The listing builds one solid part. Answer for the finished solid, in the listing's coordinates (mm). Round coordinates to 2 decimals unless told otherwise and drop trailing zeros. Write each loop counter-clockwise with the first axis right and the second up, starting at its lowest first coordinate (ties: lowest second). Pieces come first, ordered by that corner, then holes.
(1) A cutting plane is placed at B-B, the plane y = -19. Give the vertices of the cut face in (x, z), and give its area (3 significant figures).
(2) Find the intervals of material crossed by probe 1 along X at (y, z) = (-17.5, -0.25); probe 2 along Y at (x, z) = (-45, 0.5); probe 3 along Y at (x, z) = (-22.5, 1), in increasing order.
(3) A cutting plane is placed at D-D, the plane x = -21. Give the vertices of the cut face in (y, z).
(4) A cutting plane is placed at C-C, the plane z = -3.5. Give the vertices of the cut face in (x, y), and give its area (3 significant figures).
(5) A cutting plane is placed at A-A, the plane x = -44.5. Give the vertices of the cut face in (y, z), and give its area (3 significant figures).
(6) Each of these flat-tipped pins is pushed along its axis until it touches: pin 1 Ø1.5 at (y, z) = (87, -1) entering from -X; pin 2 Ø3.5 at (y, z) = (-87, -2.5) entering from +X; pin 3 Ø2 at (x, y) = (14.5, 87) entering from -Z; pin 4 Ø3.5 at (x, z) = (-9, 0) entering from +Y. Where does it stop, or does it pass through?
from build123d import *

# Parameters (mm, degrees)
SKETCH1_W           = 111
SKETCH1_H           = 178
SKETCH1_W_2         = 101
SKETCH1_H_2         = 168
BOSS_EXTRUDE1_DEPTH = 6
SKETCH2_W           = 111
SKETCH2_H           = 178
SKETCH2_W_2         = 97
SKETCH2_H_2         = 155.54954955
BOSS_EXTRUDE2_DEPTH = 0.5
SKETCH3_W           = 60
SKETCH3_H           = 10
CUT_EXTRUDE1_DEPTH  = 77
SKETCH4_W           = 65
SKETCH4_H           = 10
CUT_EXTRUDE2_DEPTH  = 77
FILLET1_R           = 1
FILLET2_R           = 3
FILLET3_R           = 1


with BuildPart() as part:
    # Sketch1 → Boss-Extrude1 (new, symmetric)
    with BuildSketch(Plane.XY):
        Rectangle(SKETCH1_W, SKETCH1_H)
        Rectangle(SKETCH1_W_2, SKETCH1_H_2, mode=Mode.SUBTRACT)
    extrude(amount=BOSS_EXTRUDE1_DEPTH, both=True)

    # Sketch2 → Boss-Extrude2 (add, symmetric)
    with BuildSketch(Plane.XY.offset(6)):
        Rectangle(SKETCH2_W, SKETCH2_H)
        Rectangle(SKETCH2_W_2, SKETCH2_H_2, mode=Mode.SUBTRACT)
    extrude(amount=BOSS_EXTRUDE2_DEPTH, both=True)

    # Sketch3 → Cut-Extrude1 (cut)
    with BuildSketch(Plane.XZ.offset(-84)):
        with Locations((0, -1)):
            Rectangle(SKETCH3_W, SKETCH3_H)
    extrude(amount=-CUT_EXTRUDE1_DEPTH, mode=Mode.SUBTRACT)

    # Sketch4 → Cut-Extrude2 (cut)
    with BuildSketch(Plane(origin=(0, -84, 0), x_dir=(1, 0, 0), z_dir=(0, 1, 0))):
        with Locations((0, 6)):
            Rectangle(SKETCH4_W, SKETCH4_H)
    extrude(amount=-CUT_EXTRUDE2_DEPTH, mode=Mode.SUBTRACT)

    # Fillet1
    fillet1_edges = [part.edges().sort_by_distance(p)[0] for p in [
        (-48.5, -77.774774775, 6),
        (48.5, -77.774774775, 6),
        (48.5, 77.774774775, 6),
        (-48.5, 77.774774775, 6),
    ]]
    fillet(fillet1_edges, radius=FILLET1_R)

    # Fillet2
    # the kernel refuses this fillet: 3 mm, written as the material it takes off along each edge
    with BuildSketch(Plane(origin=(-52.5, -86, 3.5), x_dir=(0, -1, 0), z_dir=(0, 0, 1))) as fillet2_piece_1_section:
        Polygon((0, 0), (FILLET2_R, 0), (FILLET2_R, -FILLET2_R), (0, -FILLET2_R), align=None)
    fillet2_piece_1 = extrude(amount=FILLET2_R, mode=Mode.PRIVATE)
    fillet2_piece_1 = fillet2_piece_1 - Plane(origin=(-52.5, -86, 3.5), x_dir=(0.7071067811865475, 0.7071067811865477, 0), z_dir=(0, 0, 1)) * Sphere(FILLET2_R, mode=Mode.PRIVATE)
    add(fillet2_piece_1, mode=Mode.SUBTRACT)
    with BuildSketch(Plane(origin=(-52.5, 86, 3.5), x_dir=(-1, 0, 0), z_dir=(0, 0, 1))) as fillet2_piece_2_section:
        Polygon((0, 0), (FILLET2_R, 0), (FILLET2_R, -FILLET2_R), (0, -FILLET2_R), align=None)
    fillet2_piece_2 = extrude(amount=FILLET2_R, mode=Mode.PRIVATE)
    fillet2_piece_2 = fillet2_piece_2 - Plane(origin=(-52.5, 86, 3.5), x_dir=(0.7071067811865477, -0.7071067811865474, 0), z_dir=(0, 0, 1)) * Sphere(FILLET2_R, mode=Mode.PRIVATE)
    add(fillet2_piece_2, mode=Mode.SUBTRACT)
    with BuildSketch(Plane(origin=(52.5, -86, 3.5), x_dir=(0, -1, 0), z_dir=(0, 0, 1))) as fillet2_piece_3_section:
        Polygon((0, 0), (FILLET2_R, 0), (FILLET2_R, FILLET2_R), (0, FILLET2_R), align=None)
    fillet2_piece_3 = extrude(amount=FILLET2_R, mode=Mode.PRIVATE)
    fillet2_piece_3 = fillet2_piece_3 - Plane(origin=(52.5, -86, 3.5), x_dir=(-0.7071067811865476, 0.7071067811865475, 0), z_dir=(0, 0, 1)) * Sphere(FILLET2_R, mode=Mode.PRIVATE)
    add(fillet2_piece_3, mode=Mode.SUBTRACT)
    with BuildSketch(Plane(origin=(52.5, 86, 3.5), x_dir=(0, 1, 0), z_dir=(0, 0, 1))) as fillet2_piece_4_section:
        Polygon((0, 0), (FILLET2_R, 0), (FILLET2_R, -FILLET2_R), (0, -FILLET2_R), align=None)
    fillet2_piece_4 = extrude(amount=FILLET2_R, mode=Mode.PRIVATE)
    fillet2_piece_4 = fillet2_piece_4 - Plane(origin=(52.5, 86, 3.5), x_dir=(-0.7071067811865474, -0.7071067811865477, 0), z_dir=(0, 0, 1)) * Sphere(FILLET2_R, mode=Mode.PRIVATE)
    add(fillet2_piece_4, mode=Mode.SUBTRACT)
    with BuildSketch(Plane(origin=(-55.5, -86, 6.5), x_dir=(1, 0, 0), z_dir=(0, 1, 0)), Plane(origin=(55.5, 86, 6.5), x_dir=(-1, 0, 0), z_dir=(0, -1, 0))) as fillet2_piece_5:
        with BuildLine():
            CenterArc((FILLET2_R, FILLET2_R), FILLET2_R, 180, 90)
            Line((0, FILLET2_R), (0, 0))
            Line((0, 0), (FILLET2_R, 0))
        make_face()
    extrude(amount=172, mode=Mode.SUBTRACT)
    with BuildSketch(Plane(origin=(52.5, -89, 6.5), x_dir=(0, 1, 0), z_dir=(-1, 0, 0)), Plane(origin=(-52.5, 89, 6.5), x_dir=(0, -1, 0), z_dir=(1, 0, 0))) as fillet2_piece_6:
        with BuildLine():
            CenterArc((FILLET2_R, FILLET2_R), FILLET2_R, 180, 90)
            Line((0, FILLET2_R), (0, 0))
            Line((0, 0), (FILLET2_R, 0))
        make_face()
    extrude(amount=105, mode=Mode.SUBTRACT)
    with BuildSketch(Plane(origin=(55.5, 89, -13.5), x_dir=(-1, 0, 0), z_dir=(0, 0, 1))) as fillet2_piece_7:
        with BuildLine():
            CenterArc((FILLET2_R, FILLET2_R), FILLET2_R, 180, 90)
            Line((0, FILLET2_R), (0, 0))
            Line((0, 0), (FILLET2_R, 0))
        make_face()
    extrude(amount=17, mode=Mode.SUBTRACT)
    with BuildSketch(Plane(origin=(-55.5, 89, 3.5), x_dir=(0, -1, 0), z_dir=(0, 0, -1)), Plane(origin=(55.5, -89, -13.5), x_dir=(-1, 0, 0), z_dir=(0, 0, 1)), Plane(origin=(-55.5, -89, 3.5), x_dir=(1, 0, 0), z_dir=(0, 0, -1))) as fillet2_piece_8:
        with BuildLine():
            CenterArc((FILLET2_R, -FILLET2_R), FILLET2_R, 90, 90)
            Line((0, -FILLET2_R), (0, 0))
            Line((0, 0), (FILLET2_R, 0))
        make_face()
    extrude(amount=17, mode=Mode.SUBTRACT)

    # Fillet3
    fillet3_edges = [part.edges().sort_by_distance(p)[0] for p in [
        (-30, 89, -1.25),
        (-30, 88.989491568, 3.750878781),
        (30, 88.989491568, 3.750878781),
        (30, 89, -1.25),
        (-30, 84, -1),
        (30, 84, -1),
        (0, 84, 4),
        (0, -89, -1),
        (32.5, -89, -3.5),
        (-32.5, -89, -3.5),
        (32.5, -84, -3.5),
        (-32.5, -84, -3.5),
        (0, -84, -1),
    ]]
    fillet(fillet3_edges, radius=FILLET3_R)


solid = part.part
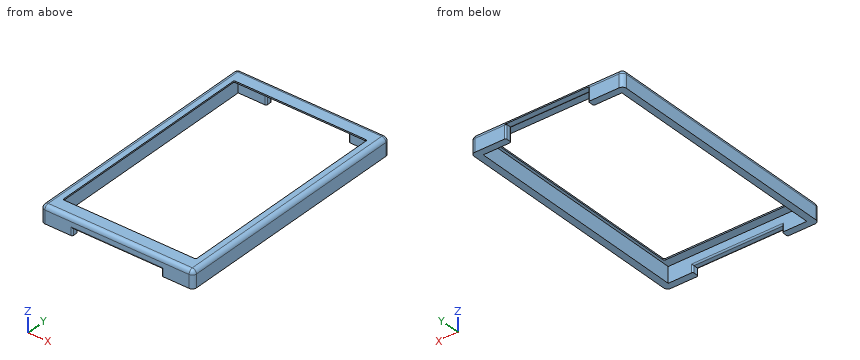
Solutions:
1. outline: (-55.5, -6) - (-50.5, -6) - (-50.5, 5.5) - (-48.5, 5.5) - (-48.5, 6.5) - (-52.5, 6.5) arc R3 ccw to (-55.5, 3.5) - close; (48.5, 5.5) - (50.5, 5.5) - (50.5, -6) - (55.5, -6) - (55.5, 3.5) arc R3 ccw to (52.5, 6.5) - (48.5, 6.5) - close
1. area: 125 mm2
2. probe 1: x = -55.5 to -50.5, 50.5 to 55.5
2. probe 2: y = -89 to -84, 84 to 89
2. probe 3: y = -89 to -84
3. outline: (-89, 0) arc R1 ccw to (-88, -1) - (-85, -1) arc R1 ccw to (-84, 0) - (-84, 5.5) - (-77.77, 5.5) - (-77.77, 6.5) - (-86, 6.5) arc R3 ccw to (-89, 3.5) - close; (77.77, 5.5) - (84, 5.5) - (84, 5) arc R1 ccw to (85, 4) - (88.96, 4) arc R3 ccw to (86, 6.5) - (77.77, 6.5) - close
4. outline: (-55.5, -86) arc R3 ccw to (-52.5, -89) - (-33.5, -89) arc R1 ccw to (-32.5, -88) - (-32.5, -85) arc R1 ccw to (-33.5, -84) - (-50.5, -84) - (-50.5, 84) - (-31, 84) arc R1 ccw to (-30, 85) - (-30, 88) arc R1 ccw to (-31, 89) - (-52.5, 89) arc R3 ccw to (-55.5, 86) - close; (30, 85) arc R1 ccw to (31, 84) - (50.5, 84) - (50.5, -84) - (33.5, -84) arc R1 ccw to (32.5, -85) - (32.5, -88) arc R1 ccw to (33.5, -89) - (52.5, -89) arc R3 ccw to (55.5, -86) - (55.5, 86) arc R3 ccw to (52.5, 89) - (31, 89) arc R1 ccw to (30, 88) - close
4. area: 2,160 mm2
5. outline: (-89, -6) - (-84, -6) - (-84, 5.5) - (-77.77, 5.5) - (-77.77, 6.5) - (-86, 6.5) arc R3 ccw to (-89, 3.5) - close; (77.77, 5.5) - (84, 5.5) - (84, -6) - (89, -6) - (89, 3.5) arc R3 ccw to (86, 6.5) - (77.77, 6.5) - close
5. area: 134 mm2
6. pin 1: stops at x = -55.49
6. pin 2: stops at x = 55.5
6. pin 3: stops at z = 4
6. pin 4: stops at y = -84
